Autodesk Inventor part; units mm, degrees
ref_plane "YZ Plane" through (0, 0, 0) normal (1, 0, 0) x (0, 1, 0)
ref_plane "XZ Plane" through (0, 0, 0) normal (0, 1, 0) x (-1, 0, 0)
ref_plane "XY Plane" through (0, 0, 0) normal (0, 0, 1) x (1, 0, 0)
sketch "Sketch1" plane through (0, 0, 0) normal (0, 1, 0) x (-1, 0, 0)
  line L0 (35, 57.25) -> (-35, 57.25)
  line L1 (-35, 57.25) -> (-35, -57.25)
  line L2 (-35, -57.25) -> (35, -57.25)
  line L3 (35, -57.25) -> (35, 57.25)
  line L4 (35, 57.25) -> (-35, -57.25) construction
  line L5 (-35, 57.25) -> (35, -57.25) construction
  point P0 (0, 0)
  dimension "d0" = 70
  dimension "d1" = 114.5
extrude "Extrusion1" add sketch "Sketch1" along normal blind 8
shell "Shell1" thickness 2 removed faces 1 at (-11.6667, 8, -19.0833)
properties part number "cap"
CAD build for the part. Positions are in the model's coordinates, mm. A direction names the side the tool comes from. Round coordinates to 2 decimals unless told otherwise and drop trailing zeros. Loops run counter-clockwise (first coordinate to the right, second up) from the corner with the lowest first, then second, coordinate; pieces in that order, holes last. Notation, with made-up numbers: M -24.5,34 L 29.5,34 A33 ccw 29.5,63 Z; hole C -29,65 d7. An arc over 180 degrees is marked long. Return JSON: item names as keys, results as strings. Group by question number.
(1) Tool access for faces 4 (the flat face through (33, 5, 1)), 5 (the flat face through (-34, 8, 17)): list every direction of +Z, -Z, +X, -X, +Y, -Y with a clear straight run to the whole face (end or side of a thin tool).
(2) Drop a flat-ended pin along its axis: P1, Ø1.5, axis at x = 4.5, z = 24.5, coming from the +Y side. Give the stop position or say it passes through.
(3) Saw through at A-A, the plane y = 4.5. List the corners of the cut face in (x, z).
(4) Saw through at B-B, the plane z = -32.5. List the corners of the cut face in (x, y).
(5) Saw through at C-C, the plane x = -20. List the corners of the cut face in (y, z).
(6) Mould opens along X. For faces 1 (the flat face through (0, 2, 1)), 2 (the flat face through (35, 4, 1)), 3 (the flat face through (0, 0, 1)) say: +X half, -X half, draft (parallel to the pull), parting line (faces both ways), or undercut.
(7) Wall check: probe 1 along Z at (x, y) = (28.5, 5.5); probe 2 along X at (y, z) = (2.25, -25); probe 3 along Y at (x, z) = (19.5, -24). Give the ranges that are in metal, low to high. Write a range as [from, to].
Answer list:
{
 "1": {"face 4": "+Y", "face 5": "+Z, -Z, +X, -X, +Y"},
 "2": {"P1": "y = 2"},
 "3": {"outline": "M -35,-57.25 L 35,-57.25 L 35,57.25 L -35,57.25 Z; hole M -33,-55.25 L 33,-55.25 L 33,55.25 L -33,55.25 Z"},
 "4": {"outline": "M -35,0 L 35,0 L 35,8 L 33,8 L 33,2 L -33,2 L -33,8 L -35,8 Z"},
 "5": {"outline": "M 0,-57.25 L 8,-57.25 L 8,-55.25 L 2,-55.25 L 2,55.25 L 8,55.25 L 8,57.25 L 0,57.25 Z"},
 "6": {"face 1": "undercut", "face 2": "+X half", "face 3": "draft"},
 "7": {"probe 1": "[-57.25, -55.25], [55.25, 57.25]", "probe 2": "[-35, -33], [33, 35]", "probe 3": "[0, 2]"}
}
